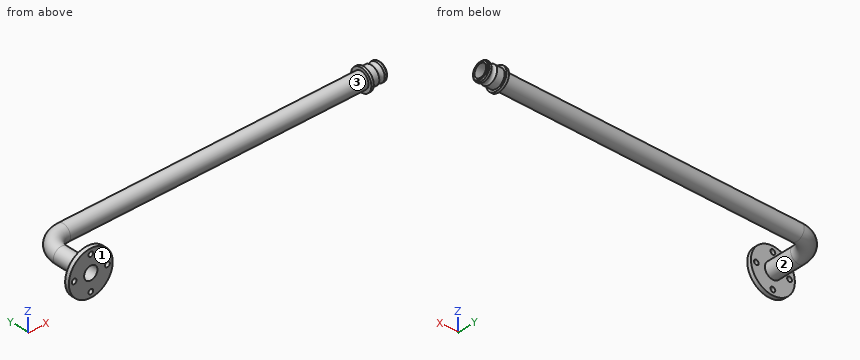
```python
from build123d import *

# Parameters (mm, degrees)
F1_R     = 30
F1_R_2   = 25
F3_R     = 82.5
F3_R_2   = 9
F3_R_3   = 25
F4_DEPTH = 15


with BuildPart() as f2:
    # F2: sweep along a path in F0
    with BuildLine(Plane.XY) as f2_path:
        Line((0, 0), (-1120, 0))
        ThreePointArc((-1120, 0), (-1176.5685424949, -23.4314575051), (-1200, -80))
        Line((-1200, -80), (-1200, -200))
    # F1 (on Right) → F2 (sweep)
    with BuildSketch(Plane.YZ):
        Circle(F1_R)
        Circle(F1_R_2, mode=Mode.SUBTRACT)
    sweep(path=f2_path.line)

    # F3 (on face) → F4 (join)
    with BuildSketch(Plane.XZ.offset(200)):
        with Locations((-1200, 0)):
            Circle(F3_R)
        with Locations((-1200, -62.5)):
            Circle(F3_R_2, mode=Mode.SUBTRACT)
        with Locations((-1262.5, 0)):
            Circle(F3_R_2, mode=Mode.SUBTRACT)
        with Locations((-1200, 0)):
            Circle(F3_R_3, mode=Mode.SUBTRACT)
        with Locations((-1137.5, 0)):
            Circle(F3_R_2, mode=Mode.SUBTRACT)
        with Locations((-1200, 62.5)):
            Circle(F3_R_2, mode=Mode.SUBTRACT)
    extrude(amount=-F4_DEPTH)

    # F5 (on Front) → F6 (revolve)
    with BuildSketch(Plane.XZ):
        with BuildLine():
            Line((0, 30), (0, 23.7858332694))
            Line((0, 23.7858332694), (69.3580582738, 23.7858332694))
            Line((69.3580582738, 23.7858332694), (69.3580582738, 30.1174111664))
            Line((69.3580582738, 30.1174111664), (65.3128772974, 33.6349532008))
            Line((65.3128772974, 33.6349532008), (57.3984086514, 33.6349532008))
            ThreePointArc((57.3984086514, 33.6349532008), (47.2854711115, 27.8227466971), (37.1725335717, 33.6349532008))
            Line((37.1725335717, 33.6349532008), (9.208066389, 33.6349532008))
            Line((9.208066389, 33.6349532008), (9.208066389, 41.5494255722))
            Line((9.208066389, 41.5494255722), (0, 41.5494255722))
            Line((0, 41.5494255722), (0, 30))
        make_face()
    revolve(axis=Axis((0, 0, 0), (-1, 0, 0)))


solid = f2.part
```
Can you work these out from the model? Positions are in its coordinate system, mm. Face numbers are marked on the shaded views. Give positions to 0.01 mm unless a question says otherwise; leave off trailing zeros. Order: outer loops, then holes, each group sorted by start corner. A loop starts at its lowest first (then second) coordinate and runs counter-clockwise, first axis right, second up. Notation, with made-up numbers: (-24, 5.5) - (-2, 5.5) arc R13 cw to (-2, 14.5) - close; hole circle Ø5 at (-2.75, 76.25). An arc over 180 degrees is marked (long way). Use a Markdown table: item, result. Add a question column.
Q1. Please list where these lines run through material, in increasing order: line 1 along Z through (x, y) = (-1200, -195); line 2 along Y through (x, z) = (-1155, -65.5); line 3 along Z through (x, y) = (-1200, -136).
Q2. If we section it at B-B on x = -744.5: Write out the boundary of the cut face in (y, z), plus the area to 3 significant figures.
Q3. I'm going to push flat-ended pins straight in: pin 1 (3 mm diameter, centred on x = -603.5, z = 24.5, fed in from -Y); pin 2 (23.5 mm diameter, centred on x = -1137.5, z = 0, fed in from +Y); pin 3 (14.5 mm diameter, centred on x = -1200, z = 62.5, fed in from -Y); pin 4 (8 mm diameter, centred on y = -20.5, z = -40, fed in from +X). Where does each tip first touch, or does it pass through?
Q4. If we mould it in two halves opening along X, with no side actions, what happens to the marked faces 1, 2 and 3? For each: released by +X, released by -X, zero draft, split by the parting line, or undercut.
Q5. If we section it at A-A on y = -143.5: Write out the boundary of the cut face in (x, z).
Answers follow:
| question | item | result |
|---|---|---|
| 1 | line 1 | z = -82.5 to -71.5, -53.5 to -25, 25 to 53.5, 71.5 to 82.5 |
| 1 | line 2 | y = -200 to -185 |
| 1 | line 3 | z = -30 to -25, 25 to 30 |
| 2 | outline | circle Ø60 at (0, 0); hole circle Ø50 at (0, 0) |
| 2 | area | 864 mm^2 |
| 3 | pin 1 | stops at y = -19.26 |
| 3 | pin 2 | stops at y = 29.85 |
| 3 | pin 3 | passes through |
| 3 | pin 4 | stops at x = 9.21 |
| 4 | face 1 | zero draft |
| 4 | face 2 | split by the parting line |
| 4 | face 3 | undercut |
| 5 | outline | circle Ø60 at (-1200, 0); hole circle Ø50 at (-1200, 0) |
